from build123d import *

# Parameters (mm, degrees)
F4_DEPTH = 25.4
F5_R     = 1.567458
F6_DEPTH = 12.7


with BuildPart() as f2:
    # F0 (on Front) → F2 (revolve)
    with BuildSketch(Plane.XZ):
        Polygon((-12.7, 0), (0, 0), (0, 20.487964), align=None)
    revolve(axis=Axis((0, 0, 41.735996), (0, 0, 1)))

    # F3 (on Top) → F4 (cut)
    with BuildSketch(Plane.XY):
        with BuildLine():
            Line((-8.870912, 10.16), (8.870912, 10.16))
            ThreePointArc((8.870912, 10.16), (0, 13.487723), (-8.870912, 10.16))
        make_face()
        with BuildLine():
            ThreePointArc((-8.870912, -10.16), (0, -13.487723), (8.870912, -10.16))
            Line((8.870912, -10.16), (-8.870912, -10.16))
        make_face()
        with BuildLine():
            ThreePointArc((10.16, -8.870912), (13.487723, 0), (10.16, 8.870912))
            Line((10.16, 8.870912), (10.16, -8.870912))
        make_face()
        with BuildLine():
            Line((-10.16, -8.870912), (-10.16, 8.870912))
            ThreePointArc((-10.16, 8.870912), (-13.487723, 0), (-10.16, -8.870912))
        make_face()
    extrude(amount=F4_DEPTH, mode=Mode.SUBTRACT)

    # F5 (on Right) → F6 (cut, symmetric)
    with BuildSketch(Plane.YZ):
        with Locations((0, 7.576898)):
            Circle(F5_R)
    extrude(amount=F6_DEPTH, both=True, mode=Mode.SUBTRACT)


solid = f2.part
For this review, take the finished solid that the model builds, in its own axes (mm). Round coordinates to 2 decimals unless told otherwise and drop trailing zeros. Order: outer loops, then holes, each group sorted by start corner. A loop starts at its lowest first (then second) coordinate and runs counter-clockwise, first axis right, second up. Notation, with made-up numbers: (82.25, -35) -> (116.25, -35) arc R25 cw to (116.25, -7) -> close; hole circle Ø9 at (-12.75, 17.5). An arc over 180 degrees is marked (long way). Put each result on its own line as item: value.
Q1. Add section A-A on z = 10.5. Write out the cut boundary in (x, y).
Check result:
outline: circle Ø12.38 at (0, 0)
Q2. Insertion check: pin 1 Ø6 at (x, z) = (2.5, 10.5) entering from -Y; pin 2 Ø4 at (x, z) = (1.5, 9.5) entering from +Y; pin 3 Ø3 at (y, z) = (5, 11) entering from +X; pin 4 Ø5 at (x, y) = (5.5, -4) entering from -Z. Each pin has a flat end and moves straight along its axis. Give the tip position at first contact, or say it passes through.
Check result:
pin 1: y = -7.8
pin 2: y = 7.95
pin 3: x = 5.22
pin 4: z = 0
Q3. Add section B-B on z = 12.75. Write out the cut boundary in (x, y), plus the area to 3 significant figures.
Check result:
outline: circle Ø9.59 at (0, 0)
area: 72.3 mm2
Q4. For probe 1 along Z at (x, y) = (4, 0); probe 2 along Z at (x, y) = (1, 0); probe 3 along Z at (x, y) = (2, 5), list the stretches that pass through material, from the lowest coordinate up. Write a range as [from, to].
Check result:
probe 1: [0, 6.01], [9.14, 14.04]
probe 2: [0, 6.01], [9.14, 18.87]
probe 3: [0, 11.8]
Q5. Mouldability with a two-part tool opening along Z and no side actions: class faces 1 (the flat face through (0, 0, 0)), 2 (the cylindrical face through (0.126, 0.723, 6.186)), 3 (the flat face through (0, -10.16, 2)) as pulls with the +Z half, pulls with the -Z half, needs draft (parallel to the pull), parting line crosses it, or undercut.
Check result:
face 1: pulls with the -Z half
face 2: undercut
face 3: needs draft
